Autodesk Inventor part; units mm, degrees
ref_plane "YZ Plane" through (0, 0, 0) normal (1, 0, 0) x (0, 1, 0)
ref_plane "XZ Plane" through (0, 0, 0) normal (0, 1, 0) x (-1, 0, 0)
ref_plane "XY Plane" through (0, 0, 0) normal (0, 0, 1) x (1, 0, 0)
sketch "Sketch1" plane through (0, 0, 0) normal (0, 1, 0) x (-1, 0, 0)
  line L0 (0, 0) -> (-16.51, 0)
  line L1 (-16.51, 0) -> (-16.51, -3.81)
  line L2 (-16.51, -3.81) -> (0, -3.81)
  line L3 (0, -3.81) -> (0, 0)
  line L4 (-16.51, 0) -> (-10.795, 0)
  line L5 (-10.795, 0) -> (-5.715, 0)
  line L6 (-5.715, 0) -> (-5.715, 2.032)
  line L7 (-5.715, 2.032) -> (-10.795, 2.032)
  line L8 (-10.795, 2.032) -> (-10.795, 0)
  line L9 (-16.51, 0) -> (-16.51, -16.51)
  line L10 (-16.51, -16.51) -> (-12.7, -16.51)
  line L11 (-12.7, -16.51) -> (-12.7, 0)
  dimension "d0" = 16.51
  dimension "d1" = 3.81
  dimension "d2" = 5.715
  dimension "d3" = 5.08
  dimension "d4" = 2.032
  dimension "d5" = 16.51
  dimension "d6" = 3.81
extrude "Extrusion1" add sketch "Sketch1" along normal blind 22.86
sketch "Sketch2" plane through (16.51, 0, 0) normal (1, 0, 0) x (0, 0, -1)
  point P0 (0, 0)
sketch "Sketch4" plane through (16.51, 0, 0) normal (1, 0, 0) x (0, 0, -1)
  line L0 (0, 0) -> (0, 22.86)
  line L1 (0, 11.43) -> (8.255, 11.43)
  dimension "d17" = 8.255
hole "Hole2" at (16.51, 11.43, -8.255) direction (-1, 0, 0) diameter 2.794 end through all
sketch "Sketch5" plane through (12.7, 0, -3.81) normal (0, 0, -1) x (-1, 0, 0)
  line L0 (0, 22.86) -> (12.7, 22.86)
  line L1 (12.7, 22.86) -> (4.445, 22.86)
  line L2 (4.445, 22.86) -> (4.445, 11.43)
  point P0 (12.7, 0)
  dimension "d46" = 8.255
  dimension "d47" = 11.43
sketch "Sketch6" plane through (12.7, 0, -3.81) normal (0, 0, -1) x (-1, 0, 0)
  point P0 (12.7, 0)
hole "Hole3" at (8.255, 11.43, -3.81) direction (0, 0, 1) diameter 5.08 end through all
properties part number "Part v4"
Input: part model. Units: mm. Frame: model coordinates. A direction names the side the tool comes from. Coordinates: 2 decimals unless noted, no trailing zeros. Write each loop counter-clockwise with the first axis right and the second up, starting at its lowest first coordinate (ties: lowest second). Pieces come first, ordered by that corner, then holes. Notation, with made-up numbers: (10.5, -2) -> (50.5, -2) arc R20 cw to (50.5, 13) -> close; hole circle Ø8 at (63.25, 72). An arc over 180 degrees is marked (long way). Write each question's results on one line, items separated by ' | '.
Item 1: Mould query, pull axis X, two halves, no side actions, for faces 6 (the flat face through (8, 18, 2.032)), 7 (the cylindrical face through (9.801, 9.414, -0.848)), 8 (the flat face through (12.7, 11, -10)). Classes: +X half, -X half, draft (parallel to the pull), parting line (faces both ways), or undercut.
Conclusion:
face 6: draft | face 7: undercut | face 8: -X half
Item 2: Material intervals for probe 1 along Z at (x, y) = (14.1, 11.43); probe 2 along X at (y, z) = (11.43, -2.35) (3 decimals); probe 3 along Z at (x, y) = (13.75, 8.75), sorted ascending.
Conclusion:
probe 1: z = -16.51 to -9.65, -6.86 to 0 | probe 2: x = 0 to 5.715, 10.795 to 16.51 | probe 3: z = -16.51 to 0
Item 3: Section query A-A on z = -8.25. Return loops of the section in (x, y), plus the area to 3 significant figures.
Conclusion:
outline: (12.7, 0) -> (16.51, 0) -> (16.51, 10.03) -> (12.7, 10.03) -> close; (12.7, 12.83) -> (16.51, 12.83) -> (16.51, 22.86) -> (12.7, 22.86) -> close | area: 76.5 mm^2
Item 4: Section query B-B on x = 6.75. Return loops of the section in (y, z).
Conclusion:
outline: (0, -3.81) -> (9.38, -3.81) -> (9.38, 2.03) -> (0, 2.03) -> close; (13.48, -3.81) -> (22.86, -3.81) -> (22.86, 2.03) -> (13.48, 2.03) -> close
Item 5: Section query C-C on y = 16. Return loops of the section in (x, z) (3 decimals).
Conclusion:
outline: (0, -3.81) -> (12.7, -3.81) -> (12.7, -16.51) -> (16.51, -16.51) -> (16.51, 0) -> (10.795, 0) -> (10.795, 2.032) -> (5.715, 2.032) -> (5.715, 0) -> (0, 0) -> close
Item 6: Section query D-D on y = 10.5. Return loops of the section in (x, z) (3 decimals).
Conclusion:
outline: (0, -3.81) -> (5.891, -3.81) -> (5.891, 2.032) -> (5.715, 2.032) -> (5.715, 0) -> (0, 0) -> close; (10.619, -3.81) -> (12.7, -3.81) -> (12.7, -7.213) -> (16.51, -7.213) -> (16.51, 0) -> (10.795, 0) -> (10.795, 2.032) -> (10.619, 2.032) -> close; (12.7, -16.51) -> (16.51, -16.51) -> (16.51, -9.297) -> (12.7, -9.297) -> close
Item 7: Set-up query: faces 1 (the flat face through (10, 0, -3)), 2 (the flat face through (14, 11, 0)), 3 (the flat face through (8, 4, 2.032)), 4 (the flat face through (5, 11, -3.81)), 5 (the flat face through (3, 11, 0)). Return all of +Z, -Z, +X, -X, +Y, -Y with unobstructed straight access to the full face (end or side cutting, diameter ignored); none if empty.
Conclusion:
face 1: +Z, -Z, +X, -X, -Y | face 2: +Z, +X, +Y, -Y | face 3: +Z, +X, -X, +Y, -Y | face 4: -Z, -X, +Y, -Y | face 5: +Z, -X, +Y, -Y
Item 8: Pin query (flat end, axial travel): pin 1 Ø1.5 at (y, z) = (10.5, -7.5) entering from -X; pin 2 Ø4.5 at (x, y) = (15, 15) entering from +Z; pin 3 Ø1.6 at (y, z) = (15.5, 1) entering from -X (3 decimals). Return the tip coordinate at first contact, or that it passes through.
Conclusion:
pin 1: stops at x = 12.7 | pin 2: stops at z = 0 | pin 3: stops at x = 5.715
